Could you check a few things on this model? Use its own coordinates, in mm. A direction names the side the tool comes from. Give positions to 0.01 mm unless a question says otherwise; leave off trailing zeros. Write each loop counter-clockwise with the first axis right and the second up, starting at its lowest first coordinate (ties: lowest second). Pieces come first, ordered by that corner, then holes. Notation, with made-up numbers: (25.5, 24) - (47.5, 24) arc R19 cw to (47.5, 58) - close; hole circle Ø3 at (71.25, -20). An arc over 180 degrees is marked (long way). Use one line per item in the form item = value.
```python
from build123d import *

# Parameters (mm, degrees)
SKETCH_1_R          = 16
EXTRUDE_1_DEPTH     = 79
SKETCH_2_R          = 4
EXTRUDE_2_DEPTH     = 14
CUT_EXTRUDE_START   = -20
SKETCH_3_R          = 16
SKETCH_3_R_2        = 15
CUT_EXTRUDE_1_DEPTH = 20
EXTRUDE_3_DEPTH     = 19
CHAMFER_1_SIZE      = 1


with BuildPart() as part:
    # 草圖1 → 填料-伸長1 (new body)
    with BuildSketch(Plane.XY):
        Circle(SKETCH_1_R)
    extrude(amount=EXTRUDE_1_DEPTH)

    # 草圖2 → 填料-伸長2 (add)
    with BuildSketch(Plane.XY.offset(79)):
        Circle(SKETCH_2_R)
    extrude(amount=EXTRUDE_2_DEPTH)

    # 草圖3 → 除料-伸長1 (cut)
    with BuildSketch(Plane.XY.offset(79).offset(CUT_EXTRUDE_START)):
        Circle(SKETCH_3_R)
        Circle(SKETCH_3_R_2, mode=Mode.SUBTRACT)
    extrude(amount=CUT_EXTRUDE_1_DEPTH, mode=Mode.SUBTRACT)

    # 草圖4 → 填料-伸長3 (add)
    with BuildSketch(Plane(origin=(0, 0, 0), x_dir=(-1, 0, 0), z_dir=(0, 0, -1))):
        with BuildLine():
            Line((14.5, 0), (14.5, 23.5))
            ThreePointArc((14.5, 23.5), (14.207106781, 24.207106781), (13.5, 24.5))
            Line((13.5, 24.5), (-13.5, 24.5))
            ThreePointArc((-13.5, 24.5), (-14.207106781, 24.207106781), (-14.5, 23.5))
            Line((-14.5, 23.5), (-14.5, 0))
            ThreePointArc((-14.5, 0), (0, -14.5), (14.5, 0))
        make_face()
    extrude(amount=EXTRUDE_3_DEPTH)

    # 導角1
    chamfer_1_edges = [part.edges().sort_by_distance(p)[0] for p in [
        (0, -14.5, -19),
        (-14.5, 11.75, -19),
        (-14.207106781, 24.207106781, -19),
        (0, 24.5, -19),
        (14.207106781, 24.207106781, -19),
        (14.5, 11.75, -19),
    ]]
    chamfer(chamfer_1_edges, length=CHAMFER_1_SIZE - 0.0001)  # a hair under: the kernel refuses the full size


solid = part.part
```
1. Which directions (+Z, -Z, +X, -X, +Y, -Y) give clear straight access to the entire face, cutting with the end or side of a thin tool? Please do faces 1 (the face through (0, 18, 0)), 2 (the face through (0, -15, 0)), 3 (the face through (-0.867, -3.905, 85.902)).
Response values:
face_1 = +Z, +Y
face_2 = -Z, -Y
face_3 = +Z
2. For pin 1 (2 mm diameter, centred on x = -11, y = 8.5, fed in from +Z); pin 2 (12 mm diameter, centred on y = 16, z = 53, fed in from -X); pin 3 (1 mm diameter, centred on x = 7, z = 29, fed in from +Y), each with a flat end and sliding along its axis, tell me the tip position at first contact or that it passes through.
Response values:
pin_1 = 79
pin_2 = -12.49
pin_3 = 14.62
3. Imagine slicing it at D-D, the plane y = 5.5. List the corners of the cut face in (x, z) for me.
Response values:
outline = (-15.02, 0) - (-14.5, 0) - (-14.5, -18) - (-13.5, -19) - (13.5, -19) - (14.5, -18) - (14.5, 0) - (15.02, 0) - (15.02, 59) - (13.96, 59) - (13.96, 79) - (-13.96, 79) - (-13.96, 59) - (-15.02, 59) - close
4. Imagine slicing it at C-C, the plane z = 40.5. List the corners of the cut face in (x, y) for me, and give its area (3 significant figures).
Response values:
outline = circle Ø32 at (0, 0)
area = 804 mm²
5. If I drill on line 1 (Z direction, x = -10, y = 3.5); line 2 (X direction, y = 15.5, z = -5); line 3 (X direction, y = 5.5, z = 49.5), over which ranges is the centre line in solid material (lowest first)? Write a range as from..to.
Response values:
line_1 = -19..79
line_2 = -14.5..14.5
line_3 = -15.02..15.02
6. Imagine slicing it at A-A, the plane x = 0. List the corners of the cut face in (y, z) for me, and give its area (3 significant figures).
Response values:
outline = (-16, 0) - (-14.5, 0) - (-14.5, -18) - (-13.5, -19) - (23.5, -19) - (24.5, -18) - (24.5, 0) - (16, 0) - (16, 59) - (15, 59) - (15, 79) - (4, 79) - (4, 93) - (-4, 93) - (-4, 79) - (-15, 79) - (-15, 59) - (-16, 59) - close
area = 3,340 mm²
7. Imagine slicing it at B-B, the plane y = 10. List the corners of the cut face in (x, z) for me.
Response values:
outline = (-14.5, -18) - (-13.5, -19) - (13.5, -19) - (14.5, -18) - (14.5, 0) - (12.49, 0) - (12.49, 59) - (11.18, 59) - (11.18, 79) - (-11.18, 79) - (-11.18, 59) - (-12.49, 59) - (-12.49, 0) - (-14.5, 0) - close
